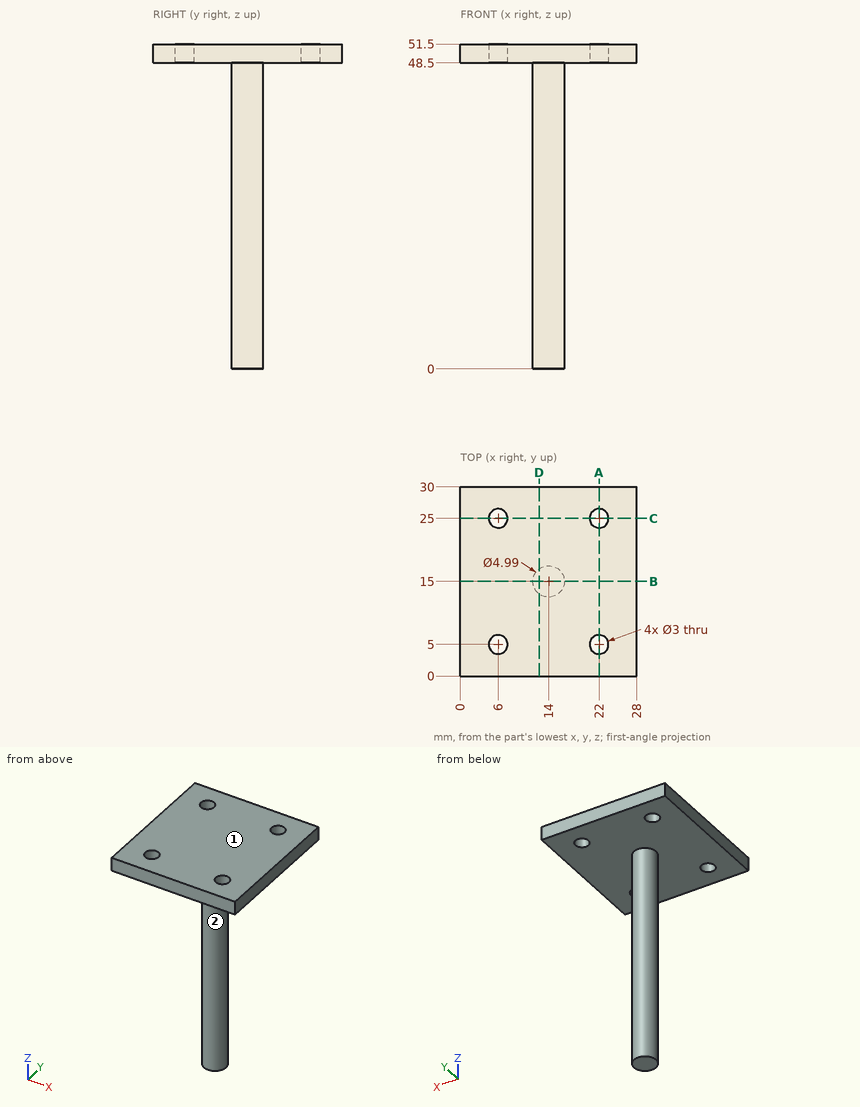
Could you check a few things on this drawing? It's one solid part, dimensions in mm from its lowest x, y, z. A direction names the side the tool comes from. Give positions to 0.01 mm unless a question says otherwise; leave off trailing zeros. Loops run counter-clockwise (first coordinate to the right, second up) from the corner with the lowest first, then second, coordinate; pieces in that order, holes last. Notation, with made-up numbers: M 32,-17 L 43,-17 A13 cw 43,-8 Z; hole C 14.25,-35.75 d4. An arc over 180 degrees is marked long. Return JSON: item names as keys, results as strings.
Item 1: Imagine slicing it at A-A on x = 22. List the corners of the cut face in (y, z) for me.
A:
{"outline": "M 0,48.5 L 3.5,48.5 L 3.5,51.5 L 0,51.5 Z; M 6.5,48.5 L 23.5,48.5 L 23.5,51.5 L 6.5,51.5 Z; M 26.5,48.5 L 30,48.5 L 30,51.5 L 26.5,51.5 Z"}
Item 2: I'm going to push flat-ended pins straight in: pin 1 Ø5 at (x, y) = (6, 5) entering from -Z; pin 2 Ø8 at (x, z) = (13, 5) entering from -Y (3 decimals). Where does each tip first touch, or does it pass through?
A:
{"pin 1": "stops at z = 48.5", "pin 2": "stops at y = 12.505"}
Item 3: Please list where these lines run through material, in increasing order: line 1 (X direction, y = 5, z = 49.6); line 2 (Y direction, x = 6, z = 50); line 3 (Z direction, x = 21, y = 13.25).
A:
{"line 1": "x = 0 to 4.5, 7.5 to 20.5, 23.5 to 28", "line 2": "y = 0 to 3.5, 6.5 to 23.5, 26.5 to 30", "line 3": "z = 48.5 to 51.5"}
Item 4: Imagine slicing it at B-B on y = 15. List the corners of the cut face in (x, z) for me (3 decimals), then the cut area to 3 significant figures.
A:
{"outline": "M 0,48.5 L 11.505,48.5 L 11.505,0 L 16.495,0 L 16.495,48.5 L 28,48.5 L 28,51.5 L 0,51.5 Z", "area": "326 mm^2"}
Item 5: Imagine slicing it at D-D on x = 12.5. List the corners of the cut face in (y, z) for me.
A:
{"outline": "M 0,48.5 L 13.01,48.5 L 13.01,0 L 16.99,0 L 16.99,48.5 L 30,48.5 L 30,51.5 L 0,51.5 Z"}
Item 6: On a 3-axis mill with a long thin cutter (end or side, diameter ignored), from which of +Z, -Z, +X, -X, +Y, -Y can I reach the whole of each face in a straight line? I mean the marked faces 1 and 2. Say none if no direction works.
A:
{"face 1": "+Z, +X, -X, +Y, -Y", "face 2": "-Z"}
Item 7: Imagine slicing it at C-C on y = 25. List the corners of the cut face in (x, z) for me.
A:
{"outline": "M 0,48.5 L 4.5,48.5 L 4.5,51.5 L 0,51.5 Z; M 7.5,48.5 L 20.5,48.5 L 20.5,51.5 L 7.5,51.5 Z; M 23.5,48.5 L 28,48.5 L 28,51.5 L 23.5,51.5 Z"}
